Could you check a few things on this model? Use its own coordinates, in mm. Face numbers are marked on the shaded views. Round coordinates to 2 decimals unless told otherwise and drop trailing zeros. Order: outer loops, then holes, each group sorted by start corner. A loop starts at its lowest first (then second) coordinate and runs counter-clockwise, first axis right, second up. Notation, with made-up numbers: (77, -30.5) - (91, -30.5) arc R20 ccw to (91, -22.5) - close; hole circle Ø9 at (36, 84). An arc over 180 degrees is marked (long way). Return JSON: item names as keys, results as strings. Group by question number.
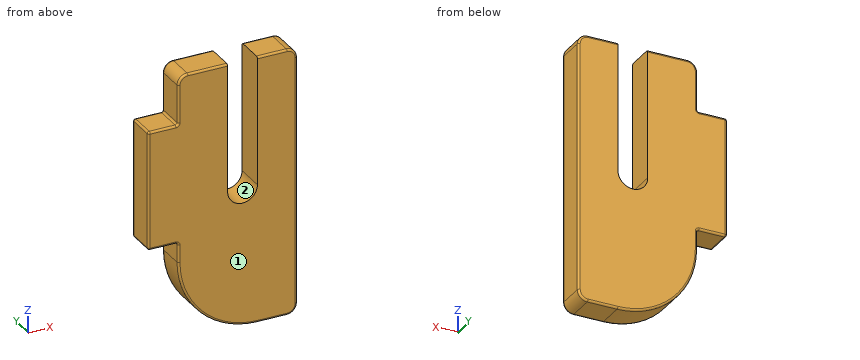
from build123d import *

# Parameters (mm, degrees)
BOSS_EXTRUDE1_DEPTH = 3
FILLET1_R           = 0.2


with BuildPart() as part:
    # Sketch1 → Boss-Extrude1 (new body)
    with BuildSketch(Plane(origin=(0, 0, 0), x_dir=(1, 0, 0), z_dir=(0, 1, 0))):
        with BuildLine():
            Line((-1.5, 0), (-1.5, -13))
            Line((-1.5, -13), (-5.5, -13))
            ThreePointArc((-5.5, -13), (-6.207106781, -12.707106781), (-6.5, -12))
            Line((-6.5, -12), (-6.5, -8))
            Line((-6.5, -8), (-9.5, -8))
            Line((-9.5, -8), (-9.5, 4))
            Line((-9.5, 4), (-6.5, 4))
            Line((-6.5, 4), (-6.5, 6))
            ThreePointArc((-6.5, 6), (-4.156854249, 11.656854249), (1.5, 14))
            Line((1.5, 14), (4.5, 14))
            ThreePointArc((4.5, 14), (5.207106781, 13.707106781), (5.5, 13))
            Line((5.5, 13), (5.5, -12))
            ThreePointArc((5.5, -12), (5.207106781, -12.707106781), (4.5, -13))
            Line((4.5, -13), (1.5, -13))
            Line((1.5, -13), (1.5, 0))
            ThreePointArc((1.5, 0), (0, 1.5), (-1.5, 0))
        make_face()
    extrude(amount=BOSS_EXTRUDE1_DEPTH)

    # Fillet1
    fillet1_edges = [part.edges().sort_by_distance(p)[0] for p in [
        (-8, 3, -4),
        (-9.5, 3, 2),
        (3, 0, -14),
        (5.207106781, 0, -13.707106781),
        (5.5, 0, -0.5),
        (5.207106781, 0, 12.707106781),
        (3, 0, 13),
        (-8, 3, 8),
        (-3.5, 0, 13),
        (-6.207106781, 0, 12.707106781),
        (-6.5, 0, 10),
        (-8, 0, 8),
        (-9.5, 0, 2),
        (-6.5, 3, 10),
        (-8, 0, -4),
        (-6.5, 0, -5),
        (-4.156854249, 0, -11.656854249),
        (-6.207106781, 3, 12.707106781),
        (-3.5, 3, 13),
        (-6.5, 1.5, 8),
        (-9.5, 1.5, 8),
        (-9.5, 1.5, -4),
        (-6.5, 1.5, -4),
        (3, 3, 13),
        (-4.156854249, 3, -11.656854249),
        (5.207106781, 3, 12.707106781),
        (5.5, 3, -0.5),
        (5.207106781, 3, -13.707106781),
        (3, 3, -14),
        (-6.5, 3, -5),
    ]]
    fillet(fillet1_edges, radius=FILLET1_R)


solid = part.part
1) We'd pull the mould along X, two halves only. Please class the marked faces 1 and 2: +X half, -X half, draft (parallel to the pull), parting line (faces both ways), or undercut.
2) I want a section at A-A, the plane y = 0.6. List the corners of the cut face in (x, z) for me.
3) If I drill on line 1 along X through (y, z) = (0.55, 8.25); line 2 along X through (y, z) = (0.8, 6.75); line 3 along Z through (x, y) = (-7.25, 2.55), over which ranges is the centre line in solid material (lowest first)? Write a range as from..to.
4) Will these pins go through, and if not, where does the flat tip stop? pin 1 (0.5 mm diameter, centred on y = 1, z = -4.5, fed in from -X); pin 2 (1.5 mm diameter, centred on x = -5, y = 0.5, fed in from -Z); pin 3 (1.5 mm diameter, centred on x = 0, y = 1, fed in from +Z).
Outcome:
{
 "1": {"face 1": "draft", "face 2": "undercut"},
 "2": {"outline": "(-9.5, -3.8) arc R0.2 ccw to (-9.3, -4) - (-6.7, -4) arc R0.2 cw to (-6.5, -4.2) - (-6.5, -6) arc R8 ccw to (1.5, -14) - (4.5, -14) arc R1 ccw to (5.5, -13) - (5.5, 12) arc R1 ccw to (4.5, 13) - (1.5, 13) - (1.5, 0) arc R1.5 cw to (-1.5, 0) - (-1.5, 13) - (-5.5, 13) arc R1 ccw to (-6.5, 12) - (-6.5, 8.2) arc R0.2 cw to (-6.7, 8) - (-9.3, 8) arc R0.2 ccw to (-9.5, 7.8) - close"},
 "3": {"line 1": "-6.5..-1.5, 1.5..5.5", "line 2": "-9.5..-1.5, 1.5..5.5", "line 3": "-4..8"},
 "4": {"pin 1": "x = -6.5", "pin 2": "z = -11.56", "pin 3": "z = -1.3"}
}
